Can you work these out from the model? Positions are in its coordinate system, mm. Face numbers are marked on the shaded views. A direction names the side the tool comes from. Give positions to 0.01 mm unless a question says otherwise; leave off trailing zeros. Order: outer loops, then holes, each group sorted by start corner. A loop starts at its lowest first (then second) coordinate and runs counter-clockwise, first axis right, second up. Notation, with made-up numbers: M 52.25,54 L 67.25,54 A13 cw 67.25,61 Z; hole C 82.5,74 d11. An arc over 180 degrees is marked long. Answer as a JSON object with one key per item and string values.
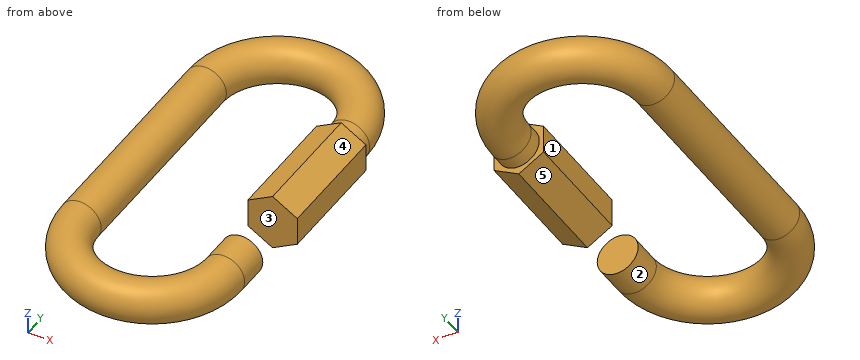
```python
from build123d import *

# Parameters (mm, degrees)
SKETCH1_R           = 3
BOSS_EXTRUDE1_DEPTH = 17


with BuildPart() as part:
    # Sweep1: sweep along a path in Sketch2
    with BuildLine(Plane.XY) as sweep1_path:
        Line((0, 0), (0, 19))
        ThreePointArc((0, 19), (-10.5, 29.5), (-21, 19))
        Line((-21, 19), (-21, -12))
        ThreePointArc((-21, -12), (-10.5, -22.5), (0, -12))
        Line((0, -12), (0, -7.5))
    # Sketch1 → Sweep1 (sweep)
    with BuildSketch(Plane(origin=(0, 0, 0), x_dir=(1, 0, 0), z_dir=(0, 1, 0))):
        Circle(SKETCH1_R)
    sweep(path=sweep1_path.line)

    # Sketch3 → Boss-Extrude1 (add)
    with BuildSketch(Plane.XZ):
        Polygon((3.623304072, 2.091915581), (0, 4.183831163), (-3.623304072, 2.091915581), (-3.623304072, -2.091915581), (0, -4.183831163), (3.623304072, -2.091915581), align=None)
    extrude(amount=-BOSS_EXTRUDE1_DEPTH)


solid = part.part
```
1) I want a section at A-A on y = 1.5. Write out the boundary of the cut face in (x, z), and give its area (3 significant figures).
Results found:
{"outline": "C -21,0 d6; M -3.62,-2.09 L 0,-4.18 L 3.62,-2.09 L 3.62,2.09 L 0,4.18 L -3.62,2.09 Z", "area": "73.8 mm²"}
2) I'm going to push flat-ended pins straight in: pin 1 Ø8 at (x, y) = (-7.5, 13.5) entering from +Z; pin 2 Ø3 at (x, z) = (-14.5, -3) entering from -Y; pin 3 Ø5 at (x, z) = (0.5, 1) entering from +Y. Where does each tip first touch, or does it pass through?
Results found:
{"pin 1": "stops at z = 2.16", "pin 2": "stops at y = -24.57", "pin 3": "stops at y = 29.39"}
3) I want a section at B-B on z = 0. Write out the boundary of the cut face in (x, y), and give its area (3 significant figures).
Results found:
{"outline": "M -24,-12 A13.5 ccw 3,-12 L 3,-7.5 L -3,-7.5 L -3,-12 A7.5 cw -18,-12 L -18,19 A7.5 cw -3,19 L -3,17 L -3.62,17 L -3.62,0 L 3.62,0 L 3.62,17 L 3,17 L 3,19 A13.5 ccw -24,19 Z", "area": "744 mm²"}
4) I need wall thicknesses on L1, parallel to X at y = 10.5, z = -0.25; L2, parallel to X at y = 1, z = -2.5; L3, parallel to Y at x = 1.25, z = 1.25. Which ranges of each line are inside material? Lowest first, please.
Results found:
{"L1": "x = -23.99 to -18.01, -3.62 to 3.62", "L2": "x = -22.66 to -19.34, -2.92 to 2.92", "L3": "y = -18.07 to -7.5, 0 to 25.07"}
5) Thinking about a two-plate mould opening in Y: for the marked faces 4 and 5, which applies, pulls with the +Y half, pulls with the -Y half, needs draft (parallel to the pull), parting line crosses it, or undercut?
Results found:
{"face 4": "needs draft", "face 5": "undercut"}
6) For the marked faces 1, 2 and 3, which set-ups out of +Z, -Z, +X, -X, +Y, -Y let a thin tool reach every point of the face, with its end or its side?
Results found:
{"face 1": "+Z, -Z", "face 2": "none", "face 3": "+Z, -Z, +X"}
